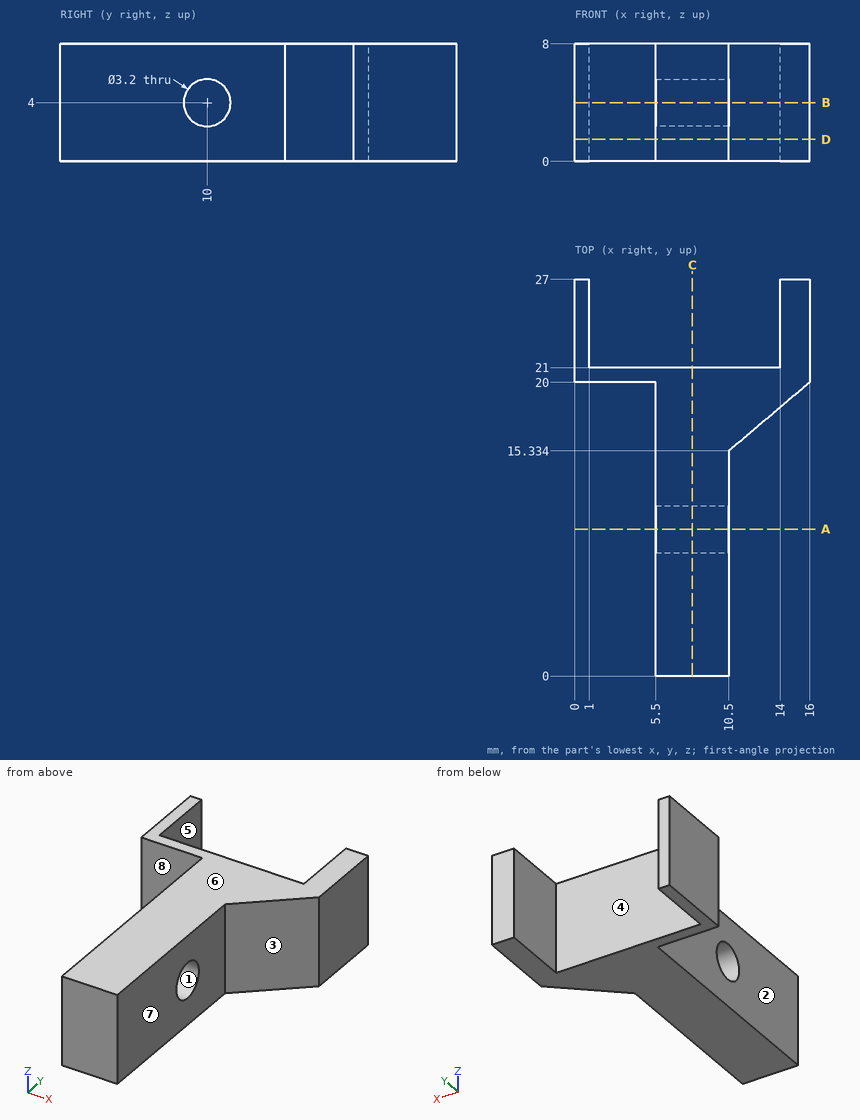
Here's the drawing with two shaded views (mm, measured from the low corner). I have some questions. A direction names the side the tool comes from. Give positions to 0.01 mm unless a question says otherwise; leave off trailing zeros. Write each loop counter-clockwise with the first axis right and the second up, starting at its lowest first coordinate (ties: lowest second). Pieces come first, ordered by that corner, then holes. Notation, with made-up numbers: (16, 71) - (52, 71) arc R21 ccw to (52, 107) - close; hole circle Ø5 at (-18.75, -29.5). An arc over 180 degrees is marked (long way). Write item = value, one per line. Start each with the question number.
1. Imagine slicing it at D-D (z = 1.5). Please give me the cut outline in (x, y).
2. On a 3-axis mill with a long thin cutter (end or side, diameter ignored), from which of +Z, -Z, +X, -X, +Y, -Y can I reach the whole of each face in a straight line? I mean the marked faces 5, 6, 7 and 8. Say none if no direction works.
3. Please list where these lines run through material, in increasing order: line 1 (Y direction, x = 9.5, z = 4); line 2 (X direction, y = 22.5, z = 7.25); line 3 (X direction, y = 4.75, z = 3.75).
4. For pin 1 (2.5 mm diameter, centred on y = 8, z = 2.5, fed in from -X); pin 2 (2.5 mm diameter, centred on x = 7.5, z = 3.5, fed in from +Y); pin 3 (1 mm diameter, centred on x = 12, z = 6, fed in from -Y), each with a flat end and sliding along its axis, tell me the tip position at first contact or that it passes through.
5. Imagine slicing it at C-C (x = 8). Please give me the cut outline in (y, z), and give its area (3 significant figures).
6. Imagine slicing it at B-B (z = 4). Please give me the cut outline in (x, y).
7. Imagine slicing it at A-A (y = 10). Please give me the cut outline in (x, z).
8. Thinking about a two-plate mould opening in Y: for the marked faces 1, 2, 3 and 4, which applies, released by +Y, released by -Y, zero draft, split by the parting line, or undercut?
Worked answers:
q1.outline = (0, 20) - (5.5, 20) - (5.5, 0) - (10.5, 0) - (10.5, 15.33) - (16, 20) - (16, 27) - (14, 27) - (14, 21) - (1, 21) - (1, 27) - (0, 27) - close
q2.face_5 = +Z, -Z, +Y
q2.face_6 = +Z, +X, -X, +Y, -Y
q2.face_7 = +Z, -Z, +X, -Y
q2.face_8 = +Z, -Z, -X, -Y
q3.line_1 = 0 to 8.4, 11.6 to 21
q3.line_2 = 0 to 1, 14 to 16
q3.line_3 = 5.5 to 10.5
q4.pin_1 = 5.5
q4.pin_2 = 21
q4.pin_3 = 16.18
q5.outline = (0, 0) - (21, 0) - (21, 8) - (0, 8) - close; hole circle Ø3.2 at (10, 4)
q5.area = 160 mm2
q6.outline = (0, 20) - (5.5, 20) - (5.5, 11.6) - (10.5, 11.6) - (10.5, 15.33) - (16, 20) - (16, 27) - (14, 27) - (14, 21) - (1, 21) - (1, 27) - (0, 27) - close; (5.5, 0) - (10.5, 0) - (10.5, 8.4) - (5.5, 8.4) - close
q7.outline = (5.5, 0) - (10.5, 0) - (10.5, 2.4) - (5.5, 2.4) - close; (5.5, 5.6) - (10.5, 5.6) - (10.5, 8) - (5.5, 8) - close
q8.face_1 = undercut
q8.face_2 = zero draft
q8.face_3 = released by -Y
q8.face_4 = released by +Y
